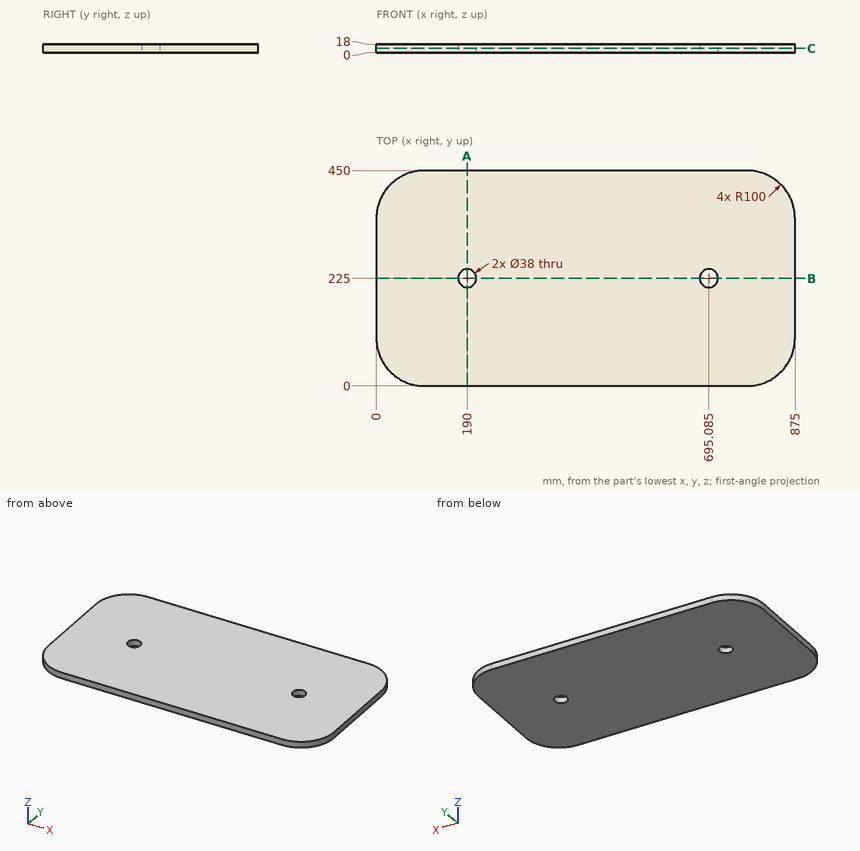
Verification items for this drawing (mm, ordinates from the low corner). Give positions to 0.01 mm unless a question says otherwise; leave off trailing zeros. Loops run counter-clockwise (first coordinate to the right, second up) from the corner with the lowest first, then second, coordinate; pieces in that order, holes last. Notation, with made-up numbers: M 26.25,76 L 77.25,76 A31 ccw 77.25,107 Z; hole C -37,86.5 d6. An arc over 180 degrees is marked long. Write item = value, one per line. Start each with the question number.
1. Thickness scan on probe 1 along X at (y, z) = (24.5, 6.75); probe 2 along X at (y, z) = (88, 6.75). Record the ranges inside material, lowest first.
2. Section check C-C, the plane z = 9. Enter the section's corners in (x, y) (1 decimal), plus the area to 3 significant figures.
3. Go/stop test with flat-tipped pins: P1, Ø10, axis at y = 79.5, z = 14.5, coming from the -X side; P2, Ø3, axis at y = 51, z = 16, coming from the +X side. Record where each tip stops, or that it passes through.
4. Section check A-A, the plane x = 190. Enter the section's corners in (y, z), plus the area to 3 significant figures.
5. Section check B-B, the plane y = 225. Enter the section's corners in (x, z) (1 decimal).
Values follow:
q1.probe_1 = 34.43 to 840.57
q1.probe_2 = 0.72 to 874.28
q2.outline = M 0,100 A100 ccw 100,0 L 775,0 A100 ccw 875,100 L 875,350 A100 ccw 775,450 L 100,450 A100 ccw 0,350 Z; hole C 190,225 d38; hole C 695.1,225 d38
q2.area = 383,000 mm^2
q3.P1 = 1.21
q3.P2 = 863
q4.outline = M 0,0 L 206,0 L 206,18 L 0,18 Z; M 244,0 L 450,0 L 450,18 L 244,18 Z
q4.area = 7,420 mm^2
q5.outline = M 0,0 L 171,0 L 171,18 L 0,18 Z; M 209,0 L 676.1,0 L 676.1,18 L 209,18 Z; M 714.1,0 L 875,0 L 875,18 L 714.1,18 Z
